Verification items for the finished model (mm, model axes). A direction names the side the tool comes from. Coordinates: 2 decimals unless noted, no trailing zeros. Order: outer loops, then holes, each group sorted by start corner. A loop starts at its lowest first (then second) coordinate and runs counter-clockwise, first axis right, second up. Notation, with made-up numbers: M 83.25,-32.75 L 93.25,-32.75 A28 cw 93.25,-10.75 Z; hole C -23.5,74 d2. An arc over 180 degrees is marked long. Return JSON: item names as keys, results as strings.
```python
from build123d import *

# Parameters (mm, degrees)
F3_R = 0.99999


# Not quite as in the source:
# - a fillet or chamfer that OpenCascade refuses, or shapes differently, is made with other operations: its cross-section is extruded or revolved along the edge and cut away or added
# - a fillet or chamfer is up to 0.001 mm smaller than in the source, because OpenCascade refuses the exact size


with BuildPart() as f1:
    # F0 (on Front) → F1 (revolve)
    with BuildSketch(Plane.XZ):
        Polygon((-23, -114.1254802332), (-27.9990236758, 45.8432773924), (-30, 45.8432773924), (-25, -114.1567226076), (-25, -154.1567226076), (-23, -154.1567226076), align=None)
    revolve(axis=Axis((0, 0, -54.1567226076), (0, 0, 1)))

    # F2: fillet of radius 100 on 2 edges, made by hand

    # F2_s1 → F2_t2 (revolve)
    with BuildSketch(Plane.XZ):
        with BuildLine():
            ThreePointArc((-25.0487923913, -112.5953660862), (-25.0121988419, -114.1569131679), (-25, -115.718841324))
            Line((-25, -115.718841324), (-25, -114.1567226076))
            Line((-25, -114.1567226076), (-25.0487923913, -112.5953660862))
        make_face()
    revolve(axis=Axis((0, 0, -114.1567226076), (0, 0, 1)))

    # F2_s3 → F2_t4 (revolve, cut)
    with BuildSketch(Plane.XZ):
        with BuildLine():
            ThreePointArc((-23.0487923913, -112.5641237119), (-23.0121988419, -114.1256707936), (-23, -115.6875989497))
            Line((-23, -115.6875989497), (-23, -114.1254802332))
            Line((-23, -114.1254802332), (-23.0487923913, -112.5641237119))
        make_face()
    revolve(axis=Axis((0, 0, -114.1254802332), (0, 0, 1)), mode=Mode.SUBTRACT)

    # F3 (radius 1 in the source; OpenCascade refuses exactly that, so slightly less here)
    f3_edges = [f1.edges().sort_by_distance(p)[0] for p in [
        (27.999024, 0, 45.843277),
        (30, 0, 45.843277),
        (25, 0, -154.156723),
        (23, 0, -154.156723),
    ]]
    fillet(f3_edges, radius=F3_R)


solid = f1.part
```
Q1. Cross-section at D-D, the plane z = -89. Record the boundary of the cut face in (x, y), and give its area (3 significant figures).
Values:
{"outline": "C 0,0 d51.57; hole C 0,0 d47.57", "area": "312 mm^2"}
Q2. Go/stop test with flat-tipped pins: pin 1 (5 mm diameter, centred on y = 3.5, z = -118, fed in from -X); pin 2 (1.5 mm diameter, centred on x = -12, z = -44, fed in from +Y); pin 3 (3 mm diameter, centred on y = -19, z = -111.5, fed in from +X). Record where each tip stops, or that it passes through.
Values:
{"pin 1": "x = -24.98", "pin 2": "y = 24.76", "pin 3": "x = 17.97"}
Q3. Cross-section at C-C, the plane z = -127.5. Record the boundary of the cut face in (x, y), and give its area (3 significant figures).
Values:
{"outline": "C 0,0 d50; hole C 0,0 d46", "area": "302 mm^2"}
Q4. Draft check along X on faces 3 (the face through (2.994, -22.804, -134.16)), 4 (the face through (-23.846, -7.509, -134.7)). Enter one of: pulls with the +X half, pulls with the -X half, needs draft (parallel to the pull), parting line crosses it, or undercut.
Values:
{"face 3": "undercut", "face 4": "parting line crosses it"}
Q5. Material ranges on line 1 along Y through (x, z) = (0, -130.5); line 2 along Y through (x, z) = (-25, 18), recorded low to high.
Values:
{"line 1": "-25 to -23, 23 to 25", "line 2": "-14.95 to -10.53, 10.53 to 14.95"}
Q6. Tool access check on faces 1 (the face through (5.96, 26.82, -34.99)), 2 (the face through (5.537, 24.936, -32.743)). Record the directions out of +Z, -Z, +X, -X, +Y, -Y that give a thin tool (end or side, any length) a straight path to the whole face; none if there is none.
Values:
{"face 1": "-Z", "face 2": "+Z"}
